```python
from build123d import *

# Parameters (mm, degrees)
F0_R     = 55
F1_DEPTH = 6
F2_R     = 42.25
F2_R_2   = 35
F3_DEPTH = 4
F5_DEPTH = 2
F6_R     = 22.5
F7_DEPTH = 6.001


with BuildPart() as f1:
    # F0 (on Top) → F1 (new body)
    with BuildSketch(Plane.XY):
        Circle(F0_R)
    extrude(amount=F1_DEPTH)

    # F2 (on face) → F3 (cut)
    with BuildSketch(Plane.XY.offset(6)):
        Circle(F2_R)
        Circle(F2_R_2, mode=Mode.SUBTRACT)
    extrude(amount=-F3_DEPTH, mode=Mode.SUBTRACT)

    # F4 (on face) → F5 (cut)
    with BuildSketch(Plane.XY.offset(6)):
        with BuildLine():
            Line((-3.5, 48.10478), (-3.5, 42.10478))
            ThreePointArc((-3.5, 42.10478), (0, 42.25), (3.5, 42.10478))
            Line((3.5, 42.10478), (3.5, 48.10478))
            ThreePointArc((3.5, 48.10478), (0, 51.60478), (-3.5, 48.10478))
        make_face()
        with BuildLine():
            Line((-48.10478, -3.5), (-42.10478, -3.5))
            ThreePointArc((-42.10478, -3.5), (-42.25, 0), (-42.10478, 3.5))
            Line((-42.10478, 3.5), (-48.10478, 3.5))
            ThreePointArc((-48.10478, 3.5), (-51.60478, 0), (-48.10478, -3.5))
        make_face()
        with BuildLine():
            Line((3.5, -48.10478), (3.5, -42.10478))
            ThreePointArc((3.5, -42.10478), (0, -42.25), (-3.5, -42.10478))
            Line((-3.5, -42.10478), (-3.5, -48.10478))
            ThreePointArc((-3.5, -48.10478), (0, -51.60478), (3.5, -48.10478))
        make_face()
        with BuildLine():
            Line((48.10478, 3.5), (42.10478, 3.5))
            ThreePointArc((42.10478, 3.5), (42.25, 0), (42.10478, -3.5))
            Line((42.10478, -3.5), (48.10478, -3.5))
            ThreePointArc((48.10478, -3.5), (51.60478, 0), (48.10478, 3.5))
        make_face()
    extrude(amount=-F5_DEPTH, mode=Mode.SUBTRACT)

    # F6 (on face) → F7 (cut, through all)
    with BuildSketch(Plane.XY.offset(6)):
        Circle(F6_R)
    extrude(amount=-F7_DEPTH, mode=Mode.SUBTRACT)


solid = f1.part
```
CAD build for the part. Positions are in the model's coordinates, mm. A direction names the side the tool comes from. Round coordinates to 2 decimals unless told otherwise and drop trailing zeros. Order: outer loops, then holes, each group sorted by start corner. A loop starts at its lowest first (then second) coordinate and runs counter-clockwise, first axis right, second up.
Q1. Two-plate mould, pull along X, no slides. Class faces 1 (the cylindrical face through (-11.923, -53.692, 2.958)), 2 (the cylindrical face through (-51.604, 0.077, 5.014)), 3 (the flat face through (-37, 21, 6)): pulls with the +X half, pulls with the -X half, needs draft (parallel to the pull), parting line crosses it, or undercut.
Q2. Slice it at B-B (x = 0). Write the cut outline in (y, z).
Q3. Which spindle directions (+Z, -Z, +X, -X, +Y, -Y) get a long thin tool onto all of the face, cutting with end or side? Do faces 4 (the cylindrical face through (10.382, -19.961, 3.042)), 5 (the flat face through (47, 0, 4)). Say none if no direction does.
Q4. Drop flat-ended pins along their axis: pin 1 (1.6 mm diameter, centred on y = -44.5, z = 5.5, fed in from -X); pin 2 (2 mm diameter, centred on x = -45, z = 5, fed in from +Y); pin 3 (2 mm diameter, centred on x = 4.5, z = 2, fed in from +Y). Give the stop position or say it passes through.
Q5. Wall check: L1, parallel to Y at x = 0, z = 3.5; L2, parallel to X at y = 26, z = 5.2; L3, parallel to X at y = 1, z = 4.8. Give the ranges that are in metal, low to high.
Q6. Slice it at D-D (x = 27). Write the cut outline in (y, z).
Q7. Slice it at A-A (z = 5.1). Write the cut outline in (x, y).
Results below:
1. face 1: parting line crosses it
1. face 2: undercut
1. face 3: needs draft
2. outline: (-55, 0) - (-22.5, 0) - (-22.5, 6) - (-35, 6) - (-35, 2) - (-42.25, 2) - (-42.25, 4) - (-51.6, 4) - (-51.6, 6) - (-55, 6) - close; (22.5, 0) - (55, 0) - (55, 6) - (51.6, 6) - (51.6, 4) - (42.25, 4) - (42.25, 2) - (35, 2) - (35, 6) - (22.5, 6) - close
3. face 4: +Z, -Z
3. face 5: +Z
4. pin 1: stops at x = -33.4
4. pin 2: stops at y = 33
4. pin 3: stops at y = 54.89
5. L1: y = -55 to -42.25, -35 to -22.5, 22.5 to 35, 42.25 to 55
5. L2: x = -48.47 to -33.3, -23.43 to 23.43, 33.3 to 48.47
5. L3: x = -54.99 to -51.46, -34.99 to -22.48, 22.48 to 34.99, 51.46 to 54.99
6. outline: (-47.92, 0) - (47.92, 0) - (47.92, 6) - (32.5, 6) - (32.5, 2) - (22.27, 2) - (22.27, 6) - (-22.27, 6) - (-22.27, 2) - (-32.5, 2) - (-32.5, 6) - (-47.92, 6) - close
7. outline: circle Ø110 at (0, 0); circle Ø70 at (0, 0); hole (-48.1, -3.5) - (-42.1, -3.5) arc R42.25 ccw to (-3.5, -42.1) - (-3.5, -48.1) arc R3.5 ccw to (3.5, -48.1) - (3.5, -42.1) arc R42.25 ccw to (42.1, -3.5) - (48.1, -3.5) arc R3.5 ccw to (48.1, 3.5) - (42.1, 3.5) arc R42.25 ccw to (3.5, 42.1) - (3.5, 48.1) arc R3.5 ccw to (-3.5, 48.1) - (-3.5, 42.1) arc R42.25 ccw to (-42.1, 3.5) - (-48.1, 3.5) arc R3.5 ccw to start; hole circle Ø45 at (0, 0)
